Check sheet for the modelled part. Datum: model origin and axes. Units: mm. A direction names the side the tool comes from. Coordinates: 2 decimals unless noted, no trailing zeros. Loops run counter-clockwise (first coordinate to the right, second up) from the corner with the lowest first, then second, coordinate; pieces in that order, holes last. Notation, with made-up numbers: M 76.5,53 L 97.5,53 A15 ccw 97.5,62 Z; hole C 20,83 d8. An arc over 180 degrees is marked long. Return JSON: item names as keys, results as strings.
from build123d import *

# Parameters (mm, degrees)
BOSS_EXTRUDE1_DEPTH = 26.7
FILLET1_R           = 4
FILLET2_R           = 1
CHAMFER1_SIZE       = 0.5
CHAMFER2_SIZE       = 0.5
SKETCH2_R           = 2
CUT_EXTRUDE1_DEPTH  = 12


with BuildPart() as part:
    # Sketch1 → Boss-Extrude1 (new body)
    with BuildSketch(Plane(origin=(0, 0, 0), x_dir=(1, 0, 0), z_dir=(0, 1, 0))):
        Polygon((10.4, 10.7), (-10.4, 10.7), (-14.4, 2.7), (-14.4, -6.7), (-12.4, -6.7), (-11.15, -10.7), (-3, -10.7), (0, -3.7), (3, -10.7), (11.15, -10.7), (12.4, -6.7), (14.4, -6.7), (14.4, 2.7), align=None)
    extrude(amount=BOSS_EXTRUDE1_DEPTH)

    # Fillet1
    fillet1_edges = [part.edges().sort_by_distance(p)[0] for p in [
        (-14.4, 13.35, -2.7),
        (-10.4, 13.35, -10.7),
        (10.4, 13.35, -10.7),
        (14.4, 13.35, -2.7),
    ]]
    fillet(fillet1_edges, radius=FILLET1_R)

    # Fillet2
    fillet2_edges = [part.edges().sort_by_distance(p)[0] for p in [
        (-3, 13.35, 10.7),
        (-11.15, 13.35, 10.7),
        (-12.4, 13.35, 6.7),
        (12.4, 13.35, 6.7),
        (11.15, 13.35, 10.7),
        (3, 13.35, 10.7),
    ]]
    fillet(fillet2_edges, radius=FILLET2_R)

    # Chamfer1
    chamfer1_edges = [part.edges().sort_by_distance(p)[0] for p in [
        (-14.4, 13.35, 6.7),
        (14.4, 13.35, 6.7),
    ]]
    chamfer(chamfer1_edges, length=CHAMFER1_SIZE)

    # Chamfer2
    chamfer2_edges = [part.edges().sort_by_distance(p)[0] for p in [
        (-13.517595457, 0, 6.7),
        (-13.517595457, 26.7, 6.7),
        (-14.4, 0, 2.222135955),
        (1.370125564, 26.7, 6.896959649),
        (14.4, 0, 2.222135955),
        (13.517595457, 0, 6.7),
        (14.15, 0, 6.45),
        (-14.15, 0, 6.45),
        (-14.4, 26.7, 2.222135955),
        (13.517595457, 26.7, 6.7),
        (14.4, 26.7, 2.222135955),
        (14.15, 26.7, 6.45),
        (-14.15, 26.7, 6.45),
        (1.370125564, 0, 6.896959649),
        (-12.741640786, 0, -6.016718427),
        (0, 0, -10.7),
        (12.741640786, 0, -6.016718427),
        (-10.030788493, 0, -10.102603233),
        (10.030788493, 0, -10.102603233),
        (14.292995958, 0, -2.674739772),
        (-14.292995958, 0, -2.674739772),
        (-12.741640786, 26.7, -6.016718427),
        (12.741640786, 26.7, -6.016718427),
        (0, 26.7, -10.7),
        (-10.030788493, 26.7, -10.102603233),
        (10.030788493, 26.7, -10.102603233),
        (14.292995958, 26.7, -2.674739772),
        (-14.292995958, 26.7, -2.674739772),
        (-1.370125564, 0, 6.896959649),
        (-1.370125564, 26.7, 6.896959649),
        (11.775, 0, 8.7),
        (7.037102622, 0, 10.7),
        (-7.037102622, 0, 10.7),
        (-11.775, 0, 8.7),
        (-11.007145565, 0, 10.505690695),
        (11.007145565, 0, 10.505690695),
        (3.108905149, 0, 10.534841092),
        (-3.108905149, 0, 10.534841092),
        (-7.037102622, 26.7, 10.7),
        (-11.775, 26.7, 8.7),
        (7.037102622, 26.7, 10.7),
        (11.775, 26.7, 8.7),
        (-11.007145565, 26.7, 10.505690695),
        (11.007145565, 26.7, 10.505690695),
        (3.108905149, 26.7, 10.534841092),
        (-3.108905149, 26.7, 10.534841092),
        (12.542854435, 0, 6.894309305),
        (12.542854435, 26.7, 6.894309305),
        (-12.542854435, 0, 6.894309305),
        (-12.542854435, 26.7, 6.894309305),
    ]]
    chamfer(chamfer2_edges, length=CHAMFER2_SIZE)

    # Sketch2 → Cut-Extrude1 (cut)
    with BuildSketch(Plane(origin=(0, 0, -10.7), x_dir=(-1, 0, 0), z_dir=(0, 0, -1))):
        with Locations((-4, 22.15)):
            Circle(SKETCH2_R)
        with Locations((4, 22.15)):
            Circle(SKETCH2_R)
        with Locations((-4, 17.75)):
            Circle(SKETCH2_R)
        with Locations((4, 17.75)):
            Circle(SKETCH2_R)
        with Locations((-4, 13.35)):
            Circle(SKETCH2_R)
        with Locations((4, 13.35)):
            Circle(SKETCH2_R)
        with Locations((-4, 8.95)):
            Circle(SKETCH2_R)
        with Locations((4, 8.95)):
            Circle(SKETCH2_R)
        with Locations((-4, 4.55)):
            Circle(SKETCH2_R)
        with Locations((4, 4.55)):
            Circle(SKETCH2_R)
    extrude(amount=-CUT_EXTRUDE1_DEPTH, mode=Mode.SUBTRACT)


solid = part.part
1) Scan lines: line 1 along Y through (x, z) = (-4, -5); line 2 along Y through (x, z) = (-2.75, -2); line 3 along X through (y, z) = (4.25, -9). Record each from-to range of solid material in increasing order. Write a range as [from, to].
Answers:
{"line 1": "[0, 2.55], [6.55, 6.95], [10.95, 11.35], [15.35, 15.75], [19.75, 20.15], [24.15, 26.7]", "line 2": "[0, 2.99], [6.11, 7.39], [10.51, 11.79], [14.91, 16.19], [19.31, 20.59], [23.71, 26.7]", "line 3": "[-11.2, -5.98], [-2.02, 2.02], [5.98, 11.2]"}
2) Draft check along X on faces 1 (the face through (12.76, 13.17, -5.98)), 2 (the face through (-11.54, 26.45, 8.61)), 3 (the face through (1.35, 13.17, 6.85)). Enter one of: +X half, -X half, draft (parallel to the pull), parting line (faces both ways), or undercut.
Answers:
{"face 1": "+X half", "face 2": "-X half", "face 3": "undercut"}
3) Go/stop test with flat-tipped pins: pin 1 Ø3.5 at (x, y) = (4, 13.35) entering from -Z; pin 2 Ø3 at (x, y) = (1.5, 14.5) entering from +Z; pin 3 Ø1 at (y, z) = (16.5, -4.5) entering from +X. Record where each tip stops, or that it passes through.
Answers:
{"pin 1": "z = 1.3", "pin 2": "z = 10.45", "pin 3": "x = 13.75"}
4) Section check B-B on z = 8. Record the cut outline in (x, y).
Answers:
{"outline": "M -11.99,0.5 L -11.47,0 L -2.39,0 L -1.84,0.5 L -1.84,26.2 L -2.39,26.7 L -11.47,26.7 L -11.99,26.2 Z; M 1.84,0.5 L 2.39,0 L 11.47,0 L 11.99,0.5 L 11.99,26.2 L 11.47,26.7 L 2.39,26.7 L 1.84,26.2 Z"}
5) Set-up check for faces 4 (the face through (-12.43, 26.4, 6.73)), 5 (the face through (4.26, 19.733, -4.784)): record each of +Z, -Z, +X, -X, +Y, -Y from which the full face is reachable in a straight line by a thin tool's end or side.
Answers:
{"face 4": "+Z, -X, +Y", "face 5": "-Z"}
